from build123d import *

# Parameters (mm, degrees)
SKETCH1_R           = 2
SKETCH1_W           = 10
SKETCH1_H           = 100
BOSS_EXTRUDE1_DEPTH = 10


with BuildPart() as part:
    # Sketch1 → Boss-Extrude1 (new body)
    with BuildSketch(Plane(origin=(0, 0, 0), x_dir=(1, 0, 0), z_dir=(0, 1, 0))):
        Polygon((-200, 530), (-200, 0), (-120, 0), (-120, 110), (113, 110), (113, 0), (200, 0), (200, 530), align=None)
        with Locations((-160, 500)):
            Circle(SKETCH1_R, mode=Mode.SUBTRACT)
        with Locations((-55, 500)):
            Circle(SKETCH1_R, mode=Mode.SUBTRACT)
        with Locations((55, 500)):
            Circle(SKETCH1_R, mode=Mode.SUBTRACT)
        with Locations((160, 500)):
            Circle(SKETCH1_R, mode=Mode.SUBTRACT)
        with Locations((-170, 50)):
            Circle(SKETCH1_R, mode=Mode.SUBTRACT)
        with Locations((-170, 260)):
            Circle(SKETCH1_R, mode=Mode.SUBTRACT)
        with Locations((-170, 440)):
            Circle(SKETCH1_R, mode=Mode.SUBTRACT)
        with Locations((170, 440)):
            Circle(SKETCH1_R, mode=Mode.SUBTRACT)
        with Locations((170, 260)):
            Circle(SKETCH1_R, mode=Mode.SUBTRACT)
        with Locations((170, 50)):
            Circle(SKETCH1_R, mode=Mode.SUBTRACT)
        with Locations((-150, 10)):
            Circle(SKETCH1_R, mode=Mode.SUBTRACT)
        with Locations((-150, 460)):
            Circle(SKETCH1_R, mode=Mode.SUBTRACT)
        with Locations((-135, 265)):
            Rectangle(SKETCH1_W, SKETCH1_H, mode=Mode.SUBTRACT)
        with Locations((120, 265)):
            Rectangle(SKETCH1_W, SKETCH1_H, mode=Mode.SUBTRACT)
    extrude(amount=BOSS_EXTRUDE1_DEPTH)


solid = part.part
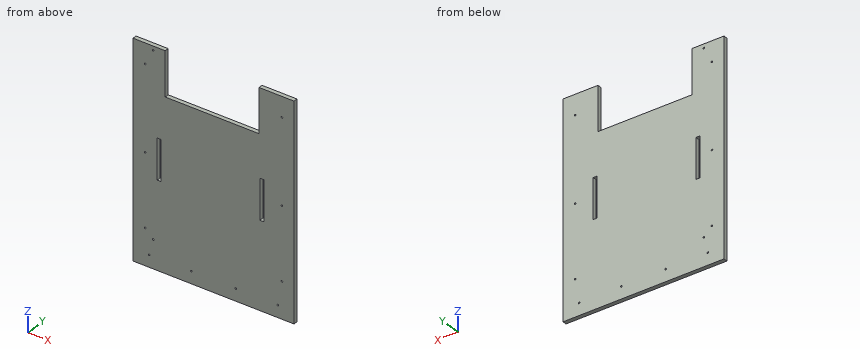
Read the model definition and answer for the solid it produces. Units are mm, in the model's axes. Give positions to 0.01 mm unless a question says otherwise; leave off trailing zeros. Write each loop counter-clockwise with the first axis right and the second up, starting at its lowest first coordinate (ties: lowest second). Pieces come first, ordered by that corner, then holes. Notation, with made-up numbers: M -12,39.5 L 44,39.5 A35 ccw 44,75.5 Z; hole C -3.5,13 d5. An arc over 180 degrees is marked long. One line per item, written item: value. Start each with the question number.
(1) Find the intervals of material crossed by line 1 (X direction, y = 4.25, z = -500); line 2 (X direction, y = 6.5, z = -10); line 3 (X direction, y = 8.25, z = -50), in increasing order.
(2) Find section B-B (x = -35.5). Determine the outline of the cut face in (y, z).
(3) A flat-ended cylindrical pin translates along its axis: pin 1 Ø3 at (x, y) = (-38, 7) entering from +Z. Find the tip coordinate at first contact, or state that the pin passes through.
(4) Find section A-A (y = 1.5). Give the number of separate pieces and of enclosed holes in the cut face, plus the area to 3 significant figures.
Results below:
1. line 1: x = -200 to -162, -158 to -57, -53 to 53, 57 to 158, 162 to 200
1. line 2: x = -200 to -152, -148 to -120, 113 to 200
1. line 3: x = -200 to -172, -168 to -120, 113 to 168, 172 to 200
2. outline: M 0,-530 L 10,-530 L 10,-110 L 0,-110 Z
3. pin 1: stops at z = -110
4. separate pieces: 1
4. enclosed holes: 14
4. area: 184,000 mm^2
